Read the model definition and answer for the solid it produces. Units are mm, in the model's axes. A direction names the side the tool comes from. Coordinates: 2 decimals unless noted, no trailing zeros. Write each loop counter-clockwise with the first axis right and the second up, starting at its lowest first coordinate (ties: lowest second). Pieces come first, ordered by that corner, then holes.
Autodesk Inventor part; units mm, degrees
ref_plane "FDT_PIRODACC_M1_XY" through (-13.5, 0, 0) normal (-1, 0, 0) x (0, 1, 0)
ref_plane "FDT_PIRODACC_M1_YZ" through (-13.5, 0, 0) normal (0, 1, 0) x (0, 0, -1)
ref_plane "FDT_PIRODACC_M1_ZX" through (-13.5, 0, 0) normal (0, 0, -1) x (-1, 0, 0)
sketch "Sketch_1" plane through (0, 0, 0) normal (0, 0, 1) x (1, 0, 0)
  line L0 (40, 0) -> (-5.5, 0)
  line L1 (-5.5, 0) -> (-5.5, 5)
  line L2 (-5.5, 5) -> (40, 5)
  line L3 (40, 5) -> (40, 0)
  line L4 (40, 0) -> (-5.5, 0)
revolve "Revolution1" add sketch "Sketch_1" angle 360 about axis through (40, 0, 0) along (1, 0, 0)
sketch "Sketch_11" plane through (0, 0, 0) normal (0, 0, 1) x (1, 0, 0)
  line L0 (40, 0) -> (35, 0)
  line L1 (35, 0) -> (35, 10)
  line L2 (35, 10) -> (40, 10)
  line L3 (40, 10) -> (40, 0)
  line L4 (40, 0) -> (35, 0)
revolve "Revolution2" add sketch "Sketch_11" angle 360 about axis through (40, 0, 0) along (1, 0, 0)
sketch "Sketch_19" plane through (0, 0, 0) normal (0, 0, 1) x (1, 0, 0)
  line L0 (-4.5, 0) -> (-21.5, 0)
  line L1 (-21.5, 0) -> (-21.5, 3.233)
  line L2 (-21.5, 3.233) -> (-20.733, 4)
  line L3 (-20.733, 4) -> (-9.4727, 4)
  line L4 (-9.4727, 4) -> (-7.0994, 3.1362)
  arc A0 (-7.0994, 3.1362) -> (-6.8942, 3.1) centre (-6.8942, 3.7) ccw
  line L5 (-6.8942, 3.1) -> (-6.1, 3.1)
  arc A1 (-6.1, 3.1) -> (-5.5, 3.7) centre (-6.1, 3.7) ccw
  line L6 (-5.5, 3.7) -> (-5.5, 4)
  line L7 (-5.5, 4) -> (-4.5, 4)
  line L8 (-4.5, 4) -> (-4.5, 0)
  line L9 (-4.5, 0) -> (-21.5, 0)
revolve "Revolution3" add sketch "Sketch_19" angle 360 about axis through (-4.5, 0, 0) along (1, 0, 0)
thread "Thread1"
sketch "Sketch_20" plane through (0, 0, 0) normal (0, 0, 1) x (1, 0, 0)
  line L0 (-32, -14.5) -> (4.4735, -14.5)
  line L1 (4.4735, -14.5) -> (-1.3, -4.5)
  line L2 (-1.3, -4.5) -> (-5.5, -4.5)
  line L3 (-5.5, -4.5) -> (-5.5, -9.5)
  line L4 (-5.5, -9.5) -> (-26.5, -9.5)
  line L5 (-26.5, -9.5) -> (-26.5, 9.5)
  line L6 (-26.5, 9.5) -> (-5.5, 9.5)
  line L7 (-5.5, 9.5) -> (-5.5, 4.5)
  line L8 (-5.5, 4.5) -> (-1.3, 4.5)
  line L9 (-1.3, 4.5) -> (4.4735, 14.5)
  line L10 (4.4735, 14.5) -> (-32, 14.5)
  line L11 (-32, 14.5) -> (-32, -14.5)
extrude "Extrusion1" cut sketch "Sketch_20" along normal mid plane 20
ref_plane "FDT_PIRODACC_M1_XY" through (-13.5, 0, 0) normal (-1, 0, 0) x (0, 1, 0)
ref_plane "FDT_PIRODACC_M1_YZ" through (-13.5, 0, 0) normal (0, 1, 0) x (0, 0, -1)
ref_plane "FDT_PIRODACC_M1_ZX" through (-13.5, 0, 0) normal (0, 0, -1) x (-1, 0, 0)
ref_plane "NUT1_XY" through (-11.5, 0, 0) normal (1, 0, 0) x (0, 0, -1)
ref_plane "NUT1_YZ" through (-11.5, 0, 0) normal (0, 0, -1) x (0, 1, 0)
ref_plane "NUT1_ZX" through (-11.5, 0, 0) normal (0, 1, 0) x (1, 0, 0)
ref_plane "PISTON_XY" through (40, 0, 0) normal (1, 0, 0) x (0, 0, -1)
ref_plane "PISTON_YZ" through (40, 0, 0) normal (0, 0, -1) x (0, 1, 0)
ref_plane "PISTON_ZX" through (40, 0, 0) normal (0, 1, 0) x (1, 0, 0)
properties part number "536233 ADN-15-P-A_(KS)"
Item 1: Given pin 1 (3 mm diameter, centred on x = -10.5, z = 0, fed in from +Y); pin 2 (6 mm diameter, centred on x = 29, z = 1.5, fed in from +Y); pin 3 (10 mm diameter, centred on x = 9, z = -8, fed in from -Y), each flat-ended and moving along its own axis, determine where each tip first touches the part or whether it passes through.
Item 2: Find the intervals of material crossed by probe 1 along X at (y, z) = (6.5, -2.5); probe 2 along X at (y, z) = (-2, -2.75); probe 3 along X at (y, z) = (-2.75, 2.5), in increasing order.
Item 3: The part is cut by section C-C (x = 28.5). Give the vertices of the cut face in (y, z), and give its area (3 significant figures).
Item 4: The part is cut by section B-B (z = 0). Give the vertices of the cut face in (x, y).
Item 5: The part is cut by section D-D (z = 8). Give the vertices of the cut face in (x, y).
Item 6: The part is cut by section A-A (y = 0). Give the vertices of the cut face in (x, z), and give its area (3 significant figures).
Item 7: Determine the mould class of faces 1 (the cylindrical face through (-6.49, 1.43, -2.75)), 2 (the flat face through (-21.5, 0, 0)), 3 (the flat face through (-3, 4.5, 0)), 4 (the flat face through (-5.5, -3.1, 2.3)) for opening direction X: +X half, -X half, draft (parallel to the pull), parting line (faces both ways), or undercut.
Item 8: For faces 5 (the cylindrical face through (37.53, -2.17, -9.76)), 6 (the cylindrical face through (15, -5, 0)), 7 (the flat face through (40, 0, 0)), 8 (the conical face through (-7.25, 1.72, -2.69)), 9 (the flat face through (-3, -4.5, 0)), determine the directions among +Z, -Z, +X, -X, +Y, -Y from which every point of the face is accessible in a straight line to the end or side of a thin tool.
Answer:
1. pin 1: stops at y = 4
1. pin 2: stops at y = 5
1. pin 3: stops at y = -4
2. probe 1: x = 35 to 40
2. probe 2: x = -21.33 to -7.83, -5.58 to 40
2. probe 3: x = -21.02 to -8.69, -5.5 to 40
3. outline: circle Ø10 at (0, 0)
3. area: 78.5 mm2
4. outline: (-21.5, -3.23) - (-20.73, -4) - (-9.47, -4) - (-7.1, -3.14) arc R0.6 cw to (-6.89, -3.1) - (-6.1, -3.1) arc R0.6 cw to (-5.5, -3.7) - (-5.5, -4.5) - (-1.3, -4.5) - (-1.01, -5) - (35, -5) - (35, -10) - (40, -10) - (40, 10) - (35, 10) - (35, 5) - (-1.01, 5) - (-1.3, 4.5) - (-5.5, 4.5) - (-5.5, 3.7) arc R0.6 cw to (-6.1, 3.1) - (-6.89, 3.1) arc R0.6 cw to (-7.1, 3.14) - (-9.47, 4) - (-20.73, 4) - (-21.5, 3.23) - close
5. outline: (35, -6) - (40, -6) - (40, 6) - (35, 6) - close
6. outline: (-21.5, -3.23) - (-20.73, -4) - (-9.47, -4) - (-7.1, -3.14) arc R0.6 cw to (-6.89, -3.1) - (-6.1, -3.1) arc R0.6 cw to (-5.5, -3.7) - (-5.5, -5) - (35, -5) - (35, -10) - (40, -10) - (40, 10) - (35, 10) - (35, 5) - (-5.5, 5) - (-5.5, 3.7) arc R0.6 cw to (-6.1, 3.1) - (-6.89, 3.1) arc R0.6 cw to (-7.1, 3.14) - (-9.47, 4) - (-20.73, 4) - (-21.5, 3.23) - close
6. area: 628 mm2
7. face 1: undercut
7. face 2: -X half
7. face 3: draft
7. face 4: undercut
8. face 5: +X, -X
8. face 6: -X
8. face 7: +Z, -Z, +X, +Y, -Y
8. face 8: none
8. face 9: +Z, -Z, -X, -Y
